Source: three-view drawing plus pictorial views. Frame: mm from the lowest corner of the part. A direction names the side the tool comes from. Coordinates: 2 decimals unless noted, no trailing zeros. Write each loop counter-clockwise with the first axis right and the second up, starting at its lowest first coordinate (ties: lowest second). Pieces come first, ordered by that corner, then holes. Notation, with made-up numbers: (62.5, 1) - (91.5, 1) arc R8 ccw to (91.5, 12) - close; hole circle Ø6 at (32.25, 72.25). An arc over 180 degrees is marked (long way). Put each result on its own line as item: value. Start each with the question number.
1. Cut plane A-A, the plane y = 20. Return loops of the section in (x, z) (1 decimal), and give its area (3 significant figures).
2. Pin query (flat end, axial travel): pin 1 (5 mm diameter, centred on x = 17, y = 8, fed in from -Z); pin 2 (8 mm diameter, centred on y = 32.5, z = 60.5, fed in from +X). Return the tip coordinate at first contact, or that it passes through.
3. Access query for the marked faces 5 and 6. Directions: +Z, -Z, +X, -X, +Y, -Y. A direction counts if a zero-diameter tool reaches every point of the face in a straight line with its end or side. Return the directions, or none.
4. Cut plane B-B, the plane z = 90. Return loops of the section in (x, y) (1 decimal).
5. Pull-direction query (X, two-part tool) for the marked faces 1, 2, 3 and 4; classes: released by +X, released by -X, zero draft, split by the parting line, or undercut.
6. Line query: line 1 (X direction, y = 20, z = 84.5) (1 decimal); line 2 (X direction, y = 11, z = 69); line 3 (Z direction, x = 42, y = 23). Output: solid intervals per line, ascending.
7. Cut plane C-C, the plane x = 63. Return loops of the section in (y, z) (1 decimal), and give its area (3 significant figures).
8. Cut plane D-D, the plane z = 7. Return loops of the section in (x, y).
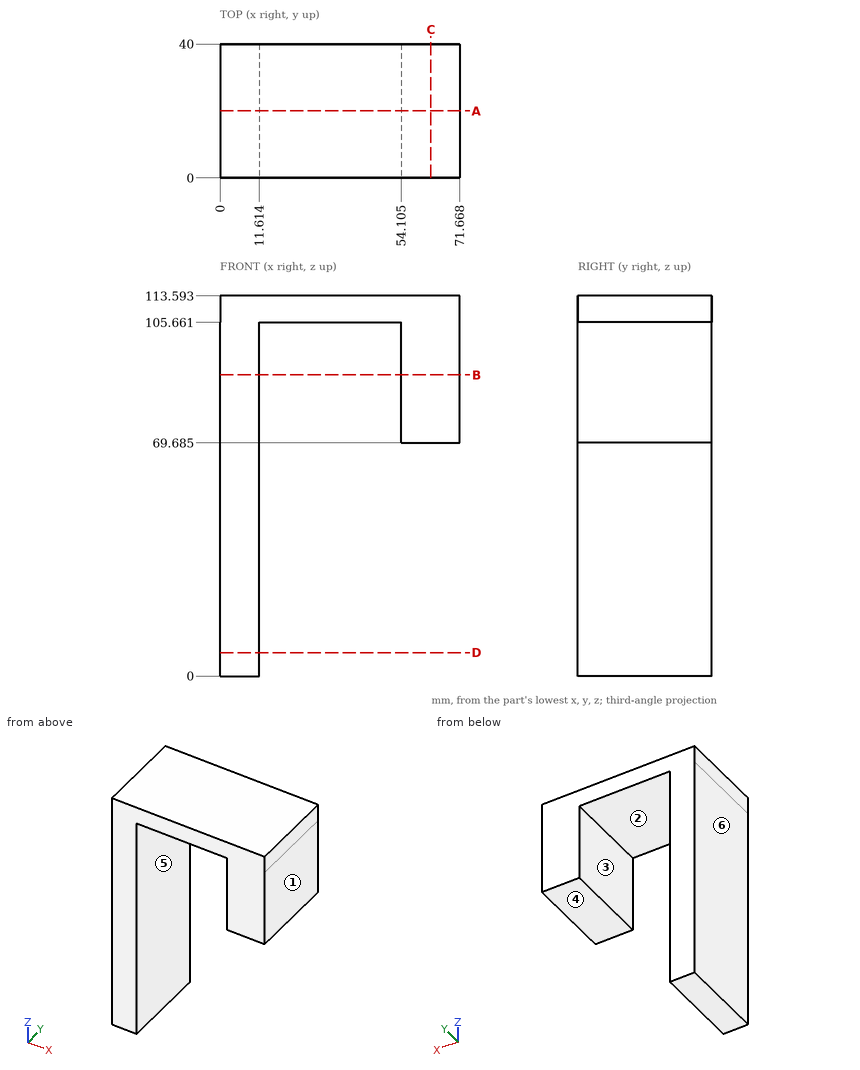
Report:
1. outline: (0, 0) - (11.6, 0) - (11.6, 105.7) - (54.1, 105.7) - (54.1, 69.7) - (71.7, 69.7) - (71.7, 113.6) - (0, 113.6) - close
1. area: 2,430 mm^2
2. pin 1: stops at z = 105.66
2. pin 2: stops at x = 11.61
3. face 5: -Z, +Y, -Y
3. face 6: +Z, -Z, -X, +Y, -Y
4. outline: (0, 0) - (11.6, 0) - (11.6, 40) - (0, 40) - close; (54.1, 0) - (71.7, 0) - (71.7, 40) - (54.1, 40) - close
5. face 1: released by +X
5. face 2: undercut
5. face 3: undercut
5. face 4: zero draft
6. line 1: x = 0 to 11.6, 54.1 to 71.7
6. line 2: x = 0 to 11.61
6. line 3: z = 105.66 to 113.59
7. outline: (0, 69.7) - (40, 69.7) - (40, 113.6) - (0, 113.6) - close
7. area: 1,760 mm^2
8. outline: (0, 0) - (11.61, 0) - (11.61, 40) - (0, 40) - close
